```python
from build123d import *

# Parameters (mm, degrees)
F0_R     = 20
F1_DEPTH = 15
F2_R     = 18
F3_DEPTH = 13
F5_R     = 3.5
F5_R_2   = 1.5
F6_DEPTH = 16
F8_DEPTH = 2


with BuildPart() as f1:
    # F0 (on Top) → F1 (new body)
    with BuildSketch(Plane.XY):
        Circle(F0_R)
    extrude(amount=F1_DEPTH)

    # F2 (on face) → F3 (cut)
    with BuildSketch(Plane.XY.offset(15)):
        Circle(F2_R)
    extrude(amount=-F3_DEPTH, mode=Mode.SUBTRACT)

    # F5 (on face) → F6 (join)
    with BuildSketch(Plane.XY.offset(2)):
        Circle(F5_R)
        Circle(F5_R_2, mode=Mode.SUBTRACT)
    extrude(amount=F6_DEPTH)

    # F7 (on Top) → F8 (cut)
    with BuildSketch(Plane.XY):
        with BuildLine():
            ThreePointArc((-16.5530215172, -7.0708895234), (-10.5801345413, -14.5623058987), (-1.6096506002, -17.9278840064))
            Line((-1.6096506002, -17.9278840064), (-3.0696488791, -4.2250092194))
            Line((-3.0696488791, -4.2250092194), (-16.5530215172, -7.0708895234))
        make_face()
        with BuildLine():
            ThreePointArc((1.6096506002, -17.9278840064), (10.5801345413, -14.5623058987), (16.5530215172, -7.0708895234))
            Line((16.5530215172, -7.0708895234), (3.0696488791, -4.2250092194))
            Line((3.0696488791, -4.2250092194), (1.6096506002, -17.9278840064))
        make_face()
        with BuildLine():
            ThreePointArc((17.5478402981, -4.0091521389), (17.8866028827, -2.0172846396), (18, 0))
            ThreePointArc((18, 0), (16.3877949898, 7.4458159641), (11.8399805143, 13.5578339502))
            Line((11.8399805143, 13.5578339502), (4.9667962199, 1.613809919))
            Line((4.9667962199, 1.613809919), (17.5478402981, -4.0091521389))
        make_face()
        with BuildLine():
            Line((0, 5.2223986007), (9.2355111332, 15.4500917184))
            ThreePointArc((9.2355111332, 15.4500917184), (0, 18), (-9.2355111332, 15.4500917184))
            Line((-9.2355111332, 15.4500917184), (0, 5.2223986007))
        make_face()
        with BuildLine():
            Line((-4.9667962199, 1.613809919), (-11.8399805143, 13.5578339502))
            ThreePointArc((-11.8399805143, 13.5578339502), (-17.1190172933, 5.5623058987), (-17.5478402981, -4.0091521389))
            Line((-17.5478402981, -4.0091521389), (-4.9667962199, 1.613809919))
        make_face()
    extrude(amount=F8_DEPTH, mode=Mode.SUBTRACT)


solid = f1.part
```
Build history of the part. All positions in model axes, mm. A direction names the side the tool comes from. Coordinates: 2 decimals unless noted, no trailing zeros. Order: outer loops, then holes, each group sorted by start corner. A loop starts at its lowest first (then second) coordinate and runs counter-clockwise, first axis right, second up. Notation, with made-up numbers: (75, -3) -> (109, -3) arc R11 cw to (109, 11) -> close; hole circle Ø9 at (78, -38). An arc over 180 degrees is marked (long way). Answer in a Markdown table with one row per item. Add a question column.
Q1. Band-saw the part on A-A, the plane z = 7.25. List the corners of the cut face in (x, y), then the cut area to 3 significant figures.
Q2. Drop flat-ended pins along their axis: pin 1 (5 mm diameter, centred on x = -2, z = 11.5, fed in from +Y); pin 2 (1.5 mm diameter, centred on x = -9, z = 6.5, fed in from +Y); pin 3 (6 mm diameter, centred on x = 9, z = 2, fed in from +Y); pin 4 (2 mm diameter, centred on x = 15.5, y = 0, fed in from -Z). Give the stop position or say it passes through.
Q3. Mould opens along Y. For faces 4 (the face through (-18, 3, 15)), 5 (the face through (8.45, 7.67, 0.99)), 6 (the face through (-4.336, -19.524, 7.395)) say: +Y half, -Y half, draft (parallel to the pull), parting line (faces both ways), or undercut.
Q4. Wall check: line 1 along Y through (x, z) = (0, 6); line 2 along X through (y, z) = (11.5, 1); line 3 along X through (y, z) = (-10.5, 1.75). Give the ranges that are in metal, low to high. Write a range as [from, to].
Q5. Band-saw the part on C-C, the plane x = 8. List the corners of the cut face in (y, z).
Q6. Band-saw the part on B-B, the plane y = 12.5. List the corners of the cut face in (x, z), then the cut area to 3 significant figures.
Q7. Which spindle directions (+Z, -Z, +X, -X, +Y, -Y) get a long thin tool onto all of the face, cutting with end or side? Do faces 1 (the face through (-11.35, -1.24, 0.99)), 2 (the face through (0, 0, 0)), 3 (the face through (3.233, -1.341, 9.888)). Say none if no direction does.
Q8. Band-saw the part on D-D, the plane y = -16. List the corners of the cut face in (x, z), then the cut area to 3 significant figures.
Answers follow:
| question | item | result |
|---|---|---|
| 1 | outline | circle Ø40 at (0, 0); circle Ø7 at (0, 0); hole circle Ø36 at (0, 0); hole circle Ø3 at (0, 0) |
| 1 | area | 270 mm^2 |
| 2 | pin 1 | y = 20 |
| 2 | pin 2 | y = 18.22 |
| 2 | pin 3 | y = 19.08 |
| 2 | pin 4 | through |
| 3 | face 4 | draft |
| 3 | face 5 | undercut |
| 3 | face 6 | parting line |
| 4 | line 1 | [-20, -18], [-3.5, -1.5], [1.5, 3.5], [18, 20] |
| 4 | line 2 | [-16.36, -13.85], [-10.66, -5.67], [5.67, 10.66], [13.85, 16.36] |
| 4 | line 3 | [-17.02, -14.62], [-2.4, 2.4], [14.62, 17.02] |
| 5 | outline | (-18.33, 0) -> (-16.12, 0) -> (-16.12, 15) -> (-18.33, 15) -> close; (-5.27, 0) -> (0.26, 0) -> (0.26, 2) -> (-5.27, 2) -> close; (6.88, 0) -> (14.08, 0) -> (14.08, 2) -> (6.88, 2) -> close; (16.12, 0) -> (18.33, 0) -> (18.33, 15) -> (16.12, 15) -> close |
| 6 | outline | (-15.61, 0) -> (-12.95, 0) -> (-12.95, 15) -> (-15.61, 15) -> close; (-11.23, 0) -> (-6.57, 0) -> (-6.57, 2) -> (-11.23, 2) -> close; (6.57, 0) -> (11.23, 0) -> (11.23, 2) -> (6.57, 2) -> close; (12.95, 0) -> (15.61, 0) -> (15.61, 15) -> (12.95, 15) -> close |
| 6 | area | 98.5 mm^2 |
| 7 | face 1 | +Z, -Z |
| 7 | face 2 | -Z, +X, -X, +Y, -Y |
| 7 | face 3 | +Z |
| 8 | outline | (-12, 0) -> (-8.25, 0) -> (-8.25, 15) -> (-12, 15) -> close; (-1.82, 0) -> (1.82, 0) -> (1.82, 2) -> (-1.82, 2) -> close; (8.25, 0) -> (12, 0) -> (12, 15) -> (8.25, 15) -> close |
| 8 | area | 120 mm^2 |
